```python
from build123d import *

# Parameters (mm, degrees)
F0_W     = 165.1
F0_H     = 127
F1_DEPTH = 9.525
F3_DEPTH = 63.5
F5_D     = 12.7
F5_DEPTH = 31.75
F5_TIP   = 3.8154649308
F7_D     = 12.7
F7_DEPTH = 31.75
F7_TIP   = 3.8154649308
F9_D     = 38.1


with BuildPart() as f1:
    # F0 (on Top) → F1 (new body)
    with BuildSketch(Plane.XY):
        with Locations((-5.9753443556, 2.5908015668)):
            Rectangle(F0_W, F0_H)
    extrude(amount=F1_DEPTH)

    # F2 (on face) → F3 (join)
    with BuildSketch(Plane.XY.offset(9.525)):
        with BuildLine():
            Line((-37.7253443556, 66.0908015668), (-88.5253443556, 66.0908015668))
            Line((-88.5253443556, 66.0908015668), (-88.5253443556, 15.2908015668))
            Line((-88.5253443556, 15.2908015668), (-63.1253443556, 15.2908015668))
            ThreePointArc((-63.1253443556, 15.2908015668), (-45.1648321135, 22.7302893247), (-37.7253443556, 40.6908015668))
            Line((-37.7253443556, 40.6908015668), (-37.7253443556, 66.0908015668))
        make_face()
        with BuildLine():
            Line((76.5746556444, 66.0908015668), (25.7746556444, 66.0908015668))
            Line((25.7746556444, 66.0908015668), (25.7746556444, 40.6908015668))
            ThreePointArc((25.7746556444, 40.6908015668), (33.2141434022, 22.7302893247), (51.1746556444, 15.2908015668))
            Line((51.1746556444, 15.2908015668), (76.5746556444, 15.2908015668))
            Line((76.5746556444, 15.2908015668), (76.5746556444, 66.0908015668))
        make_face()
    extrude(amount=F3_DEPTH)

    # F5
    with Locations(Plane.XY.offset(73.025)):
        with Locations((-63.1253443556, 40.6908015668)):
            Hole(F5_D / 2, depth=F5_DEPTH)
            with Locations((0, 0, -(F5_DEPTH + F5_TIP / 2))):  # 118° drill point
                Cone(0, F5_D / 2, F5_TIP, mode=Mode.SUBTRACT)

    # F7
    with Locations(Plane.XY.offset(73.025)):
        with Locations((51.1746556444, 40.6908015668)):
            Hole(F7_D / 2, depth=F7_DEPTH)
            with Locations((0, 0, -(F7_DEPTH + F7_TIP / 2))):  # 118° drill point
                Cone(0, F7_D / 2, F7_TIP, mode=Mode.SUBTRACT)

    # F9 (through all)
    with Locations(Plane.XY.offset(9.525)):
        with Locations((-5.9753443556, 0)):
            Hole(F9_D / 2)


solid = f1.part
```
Can you work these out from the model? Positions are in its coordinate system, mm. A direction names the side the tool comes from. Give positions to 0.01 mm unless a question says otherwise; leave off trailing zeros. Loops run counter-clockwise (first coordinate to the right, second up) from the corner with the lowest first, then second, coordinate; pieces in that order, holes last. Notation, with made-up numbers: M 80.5,72 L 99.5,72 A6 ccw 99.5,81 Z; hole C 30.25,87.25 d8. An arc over 180 degrees is marked long. One line per item, written item: value.
(1) I need wall thicknesses on line 1 (X direction, y = 47, z = 31); line 2 (Z direction, x = 70, y = -55) (3 decimals); line 3 (Y direction, x = 58, z = 51.5). Which ranges of each line are inside material? Lowest first, please.
Returned:
line 1: -88.53 to -37.73, 25.77 to 76.57
line 2: 0 to 9.525
line 3: 15.29 to 66.09
(2) Will these pins go through, and if not, where does the flat tip stop? pin 1 (4 mm diameter, centred on x = 33, z = 18.5, fed in from -Y); pin 2 (8 mm diameter, centred on x = 34, z = 30, fed in from -Y).
Returned:
pin 1: y = 21.11
pin 2: y = 18.97
(3) Which directions (+Z, -Z, +X, -X, +Y, -Y) give clear straight access to the entire face, cutting with the end or side of a thin tool? Please do faces 1 (the face through (-56.78, 40.97, 56.93)), 2 (the face through (-45.4, 22.5, 40.8)), 3 (the face through (-76, 15.291, 41)).
Returned:
face 1: +Z
face 2: +Z, -Y
face 3: +Z, +X, -X, -Y
(4) Suppose I cut it at D-D on y = 0. List the corners of the cut face in (x, z) for me (3 decimals).
Returned:
outline: M -88.525,0 L -25.025,0 L -25.025,9.525 L -88.525,9.525 Z; M 13.075,0 L 76.575,0 L 76.575,9.525 L 13.075,9.525 Z
(5) Suppose I cut it at C-C on x = -1. List the corners of the cut face in (y, z) for me (3 decimals).
Returned:
outline: M -60.909,0 L -18.389,0 L -18.389,9.525 L -60.909,9.525 Z; M 18.389,0 L 66.091,0 L 66.091,9.525 L 18.389,9.525 Z
(6) We'd pull the mould along X, two halves only. Please class faces 4 (the face through (64, 15.291, 41)), 5 (the face through (-88.525, 32, 36)), 6 (the face through (33.018, 22.929, 40.83)), 7 (the face through (50.3, 40.02, 38.12)): released by +X, released by -X, zero draft, split by the parting line, or undercut.
Returned:
face 4: zero draft
face 5: released by -X
face 6: undercut
face 7: undercut
(7) Suppose I cut it at B-B on z = 59.5. List the corners of the cut face in (x, y) for me.
Returned:
outline: M -88.53,15.29 L -63.13,15.29 A25.4 ccw -37.73,40.69 L -37.73,66.09 L -88.53,66.09 Z; M 25.77,40.69 A25.4 ccw 51.17,15.29 L 76.57,15.29 L 76.57,66.09 L 25.77,66.09 Z; hole C -63.13,40.69 d12.7; hole C 51.17,40.69 d12.7
(8) Suppose I cut it at A-A on z = 13.5. List the corners of the cut face in (x, y) for me.
Returned:
outline: M -88.53,15.29 L -63.13,15.29 A25.4 ccw -37.73,40.69 L -37.73,66.09 L -88.53,66.09 Z; M 25.77,40.69 A25.4 ccw 51.17,15.29 L 76.57,15.29 L 76.57,66.09 L 25.77,66.09 Z
